from build123d import *

# Parameters (mm, degrees)
F2_R     = 29.922306
F2_R_2   = 2
F3_DEPTH = 2.001


with BuildPart() as f1:
    # F0 (on Front) → F1 (revolve)
    with BuildSketch(Plane.XZ):
        with BuildLine():
            Line((13.5, 16), (9.798011, 16))
            ThreePointArc((9.798011, 16), (5.500023, 19.677756), (0, 21))
            Line((0, 21), (0, 0))
            Line((0, 0), (25, 0))
            Line((25, 0), (25, 2))
            Line((25, 2), (13.5, 2))
            Line((13.5, 2), (13.5, 16))
        make_face()
    revolve(axis=Axis((0, 0, 10.5), (0, 0, -1)))

    # F2 (on face) → F3 (cut, through all)
    with BuildSketch(Plane.XY.offset(2)):
        Circle(F2_R)
        with BuildLine():
            ThreePointArc((-25, 0), (-24.336437, 2.489038), (-22.521875, 4.317424))
            Line((-22.521875, 4.317424), (-7.609758, 13.027826))
            ThreePointArc((-7.609758, 13.027826), (-3.941785, 14.563481), (0, 15.0875))
            ThreePointArc((0, 15.0875), (3.941785, 14.563481), (7.609758, 13.027826))
            Line((7.609758, 13.027826), (22.521875, 4.317424))
            ThreePointArc((22.521875, 4.317424), (24.336437, 2.489038), (25, 0))
            ThreePointArc((25, 0), (24.336437, -2.489038), (22.521875, -4.317424))
            Line((22.521875, -4.317424), (7.609758, -13.027826))
            ThreePointArc((7.609758, -13.027826), (3.941785, -14.563481), (0, -15.0875))
            ThreePointArc((0, -15.0875), (-3.941785, -14.563481), (-7.609758, -13.027826))
            Line((-7.609758, -13.027826), (-22.521875, -4.317424))
            ThreePointArc((-22.521875, -4.317424), (-24.336437, -2.489038), (-25, 0))
        make_face(mode=Mode.SUBTRACT)
        with Locations((-20, 0)):
            Circle(F2_R_2)
        with Locations((20, 0)):
            Circle(F2_R_2)
    extrude(amount=-F3_DEPTH, mode=Mode.SUBTRACT)


solid = f1.part
Read the model definition and answer for the solid it produces. Units are mm, in the model's axes. A direction names the side the tool comes from. Coordinates: 2 decimals unless noted, no trailing zeros. Order: outer loops, then holes, each group sorted by start corner. A loop starts at its lowest first (then second) coordinate and runs counter-clockwise, first axis right, second up. Notation, with made-up numbers: M 62,46 L 104,46 A35 cw 104,85 Z; hole C 77.25,-39.5 d3. An arc over 180 degrees is marked long. Put each result on its own line as item: value. Start each with the question number.
Item 1: Section C-C, the plane z = 11.5 is taken. Determine the outline of the cut face in (x, y).
Item 2: Section A-A, the plane x = 20 is taken. Determine the outline of the cut face in (y, z).
Item 3: Given pin 1 Ø8 at (x, z) = (-9, 5.5) entering from +Y; pin 2 Ø5 at (y, z) = (-5, 16) entering from +X; pin 3 Ø8 at (x, z) = (4, 17) entering from -Y, each flat-ended and moving along its own axis, determine where each tip first touches the part or whether it passes through.
Item 4: Section B-B, the plane y = -1.5 is taken. Count the separate pieces of the cut face and the enclosed holes in it, plus the area to 3 significant figures.
Item 5: For faces 1 (the face through (-7.1, -7.1, 16)), 2 (the face through (15.17, -8.61, 1.01)), determine the directions among +Z, -Z, +X, -X, +Y, -Y from which every point of the face is accessible in a straight line to the end or side of a thin tool.
Item 6: The mould has two halves that part along Y. Classify faces 3 (the face through (18.4, -1.2, 1)), 4 (the face through (-2.93, 13.18, 9.1)), 5 (the face through (14.961, 8.734, 1.014)): +Y half, -Y half, draft (parallel to the pull), parting line (faces both ways), or undercut.
Item 7: Consider probe 1 along Z at (x, y) = (-7.5, 10.5); probe 2 along Y at (x, z) = (-20, 0.4); probe 3 along X at (y, z) = (1, 18.25). Determine where each line is inside the solid, lowest interval first. Write a range as [from, to].
Computed:
1. outline: C 0,0 d27
2. outline: M -5.79,0 L -2,0 L -2,2 L -5.79,2 Z; M 2,0 L 5.79,0 L 5.79,2 L 2,2 Z
3. pin 1: stops at y = 13.33
3. pin 2: stops at x = 13.27
3. pin 3: stops at y = -13.5
4. separate pieces: 3
4. enclosed holes: 0
4. area: 531 mm2
5. face 1: +Z
5. face 2: +Z, -Z, +X, -Y
6. face 3: undercut
6. face 4: parting line
6. face 5: +Y half
7. probe 1: z = [0, 16]
7. probe 2: y = [-5.79, -2], [2, 5.79]
7. probe 3: x = [-7.61, 7.61]
